```python
from build123d import *

# Parameters (mm, degrees)
SKETCH1_R           = 1.5
BOSS_EXTRUDE1_DEPTH = 3.175
CUT_EXTRUDE2_DEPTH  = 10
SKETCH6_W           = 2.65
SKETCH6_H           = 3.175
CUT_EXTRUDE3_DEPTH  = 0.25


with BuildPart() as part:
    # Sketch1 → Boss-Extrude1 (new body)
    with BuildSketch(Plane(origin=(0, 0, 0), x_dir=(1, 0, 0), z_dir=(0, 1, 0))):
        Polygon((0, 7.5), (0, 0), (444.5, 0), (444.5, 15), (0, 15), align=None)
        with Locations(Location((2.5, 2.5, 0), (0, 0, 270))):
            Circle(SKETCH1_R, mode=Mode.SUBTRACT)
        with Locations(Location((12.5, 2.5, 0), (0, 0, 270))):
            Circle(SKETCH1_R, mode=Mode.SUBTRACT)
        with Locations(Location((127.2, 2.5, 0), (0, 0, 270))):
            Circle(SKETCH1_R, mode=Mode.SUBTRACT)
        with Locations(Location((137.2, 2.5, 0), (0, 0, 270))):
            Circle(SKETCH1_R, mode=Mode.SUBTRACT)
        with Locations(Location((2.5, 12.5, 0), (0, 0, 270))):
            Circle(SKETCH1_R, mode=Mode.SUBTRACT)
        with Locations(Location((12.5, 12.5, 0), (0, 0, 270))):
            Circle(SKETCH1_R, mode=Mode.SUBTRACT)
        with Locations(Location((127.2, 12.5, 0), (0, 0, 270))):
            Circle(SKETCH1_R, mode=Mode.SUBTRACT)
        with Locations(Location((137.2, 12.5, 0), (0, 0, 270))):
            Circle(SKETCH1_R, mode=Mode.SUBTRACT)
        with Locations(Location((171.45, 7.5, 0), (0, 0, 270))):
            Circle(SKETCH1_R, mode=Mode.SUBTRACT)
        with Locations(Location((273.05, 7.5, 0), (0, 0, 270))):
            Circle(SKETCH1_R, mode=Mode.SUBTRACT)
        with Locations(Location((442, 12.5, 0), (0, 0, 270))):
            Circle(SKETCH1_R, mode=Mode.SUBTRACT)
        with Locations(Location((307.3, 2.5, 0), (0, 0, 270))):
            Circle(SKETCH1_R, mode=Mode.SUBTRACT)
        with Locations(Location((317.3, 2.5, 0), (0, 0, 270))):
            Circle(SKETCH1_R, mode=Mode.SUBTRACT)
        with Locations(Location((432, 2.5, 0), (0, 0, 270))):
            Circle(SKETCH1_R, mode=Mode.SUBTRACT)
        with Locations(Location((442, 2.5, 0), (0, 0, 270))):
            Circle(SKETCH1_R, mode=Mode.SUBTRACT)
        with Locations(Location((307.3, 12.5, 0), (0, 0, 270))):
            Circle(SKETCH1_R, mode=Mode.SUBTRACT)
        with Locations(Location((317.3, 12.5, 0), (0, 0, 270))):
            Circle(SKETCH1_R, mode=Mode.SUBTRACT)
        with Locations(Location((432, 12.5, 0), (0, 0, 270))):
            Circle(SKETCH1_R, mode=Mode.SUBTRACT)
    extrude(amount=BOSS_EXTRUDE1_DEPTH)

    # Sketch4 → Cut-Extrude2 (cut)
    with BuildSketch(Plane(origin=(0, 3.175, 0), x_dir=(1, 0, 0), z_dir=(0, 1, 0))):
        Polygon((444.5, 5.75), (444.5, 7.5), (440.5, 7.5), (440.25, 7.5), (440.25, 4.6), (442.45, 4.6), (442.45, 5.75), align=None)
        Polygon((440.5, 7.5), (444.5, 7.5), (444.5, 9), (442.2, 9), (442.2, 10.15), (440.5, 10.15), align=None)
        Polygon((2.05, 9.25), (0, 9.25), (0, 5.75), (2.05, 5.75), (2.05, 4.6), (4.25, 4.6), (4.25, 7.5), (4.25, 10.4), (2.05, 10.4), align=None)
    extrude(amount=-CUT_EXTRUDE2_DEPTH, mode=Mode.SUBTRACT)

    # Sketch6 → Cut-Extrude3 (cut)
    with BuildSketch(Plane(origin=(440.5, 0, 0), x_dir=(0, 0, -1), z_dir=(1, 0, 0))):
        with Locations((8.825, 1.5875)):
            Rectangle(SKETCH6_W, SKETCH6_H)
    extrude(amount=-CUT_EXTRUDE3_DEPTH, mode=Mode.SUBTRACT)


solid = part.part
```
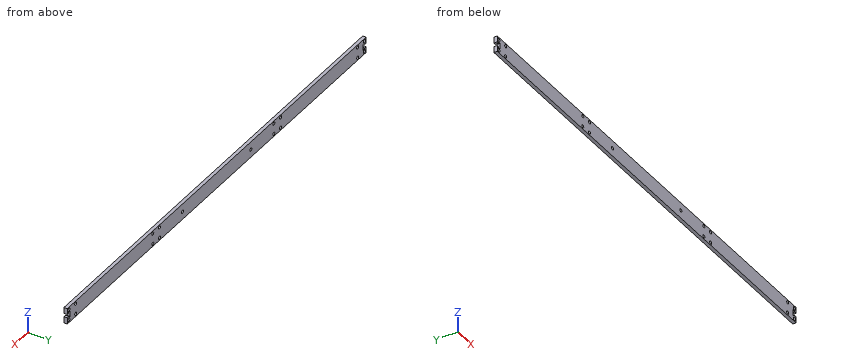
Geometry check sheet. Reference: the model listing, model coordinates, mm. Round coordinates to 2 decimals unless told otherwise and drop trailing zeros. Write item = value, one per line.
Q1. Section check A-A (y = 2.65). Give the number of separate pieces and of enclosed holes in the cut face, plus the area to 3 significant figures.
Answer block:
separate_pieces = 1
enclosed_holes = 18
area = 6,500 mm^2
Q2. Scan lines: line 1 (X direction, y = 1.75, z = -7.5); line 2 (Z direction, x = 307.3, y = 1.95). Record each from-to range of solid material in increasing order.
Answer block:
line_1 = 4.25 to 169.95, 172.95 to 271.55, 274.55 to 440.25
line_2 = -15 to -14, -11 to -4, -1 to 0
Q3. Depth check by flat-ended pin: pin 1 Ø2.5 at (x, z) = (171.45, -7.5) entering from +Y. Enter the tip coordinate at first touch or a pass-through.
Answer block:
pin_1 = through
